Read the model definition and answer for the solid it produces. Units are mm, in the model's axes. A direction names the side the tool comes from. Give positions to 0.01 mm unless a question says otherwise; leave off trailing zeros. Write each loop counter-clockwise with the first axis right and the second up, starting at its lowest first coordinate (ties: lowest second). Pieces come first, ordered by that corner, then holes. Notation, with made-up numbers: M -38,42.25 L 9,42.25 A18 ccw 9,67.25 Z; hole C 71,38.5 d3. An arc over 180 degrees is marked long. Write each question's results on one line, items separated by ' | '. Start each with the question number.
```python
from build123d import *

# Parameters (mm, degrees)
BOTTOM_COVER_SKETCH_01_W                   = 44.37
BOTTOM_COVER_SKETCH_01_H                   = 23.06
BOTTOM_COVER_EXT_SHAPE_DEPTH               = 4.3
SALIENTE_EXTRUIR1_DEPTH                    = 1.4
CORTAR_EXTRUIR1_DEPTH                      = 30.966091253
CORTAR_EXTRUIR1_DEPTH_BACK                 = 30.966091253
VACIADO2_START                             = 0.5
VACIADO2_OUTLINE_W                         = 42.97
VACIADO2_OUTLINE_H                         = 21.06
VACIADO2_DEPTH                             = 3.8
SALIENTE_EXTRUIR2_DEPTH                    = 1.4
CORTAR_EXTRUIR2_DEPTH                      = 30.933277886
CORTAR_EXTRUIR2_DEPTH_BACK                 = 30.933277886
BOTTOM_POWER_TAKE_OFF_SHAFT_SKETCH_R       = 3
POWER_TAKE_OFF_SHAFT_EXTRUDE_01_DEPTH      = 3.9
BOTTOM_POWER_TAKE_OFF_SHAFT_SKETCH_3_R     = 4
BOTTOM_POWER_TAKE_OFF_SHAFT_SKETCH_3_R_2   = 3
POWER_TAKE_OFF_SHAFT_EXTRUDE_02_DEPTH      = 1
POWER_TAKE_OFF_SHAFT_CUT_DEPTH             = 1
POWER_TAKE_OFF_SHAFT_BOTTOM_COVER_SKETCH_R = 1
CORTAR_EXTRUIR4_DEPTH                      = 4.2
REDONDEO1_R                                = 0.5


with BuildPart() as part:
    # bottom-cover-sketch-01 → Bottom-cover-ext-shape (new body)
    with BuildSketch(Plane(origin=(0, 0, 0), x_dir=(1, 0, 0), z_dir=(0, 1, 0))):
        Rectangle(BOTTOM_COVER_SKETCH_01_W, BOTTOM_COVER_SKETCH_01_H)
    extrude(amount=BOTTOM_COVER_EXT_SHAPE_DEPTH)

    # bottom-cover-sketch-01<31> → Saliente-Extruir1 (add)
    with BuildSketch(Plane(origin=(0, 0, 0), x_dir=(1, 0, 0), z_dir=(0, 1, 0))):
        with BuildLine():
            Line((4.447, 8.15), (16.025784389, 8.15))
            ThreePointArc((16.025784389, 8.15), (17.087381076, 6.195438755), (19, 5.06001547))
            Line((19, 5.06001547), (19, -5.06001547))
            ThreePointArc((19, -5.06001547), (17.087381076, -6.195438755), (16.025784389, -8.15))
            Line((16.025784389, -8.15), (4.447, -8.15))
            Line((4.447, -8.15), (4.447, 8.15))
        make_face()
    extrude(amount=-SALIENTE_EXTRUIR1_DEPTH)

    # Croquis3 → Cortar-Extruir1 (cut, two sides: drawn at the far end of the back side and taken through both)
    with BuildSketch(Plane.XY.offset(8.15).offset(-CORTAR_EXTRUIR1_DEPTH_BACK)):
        Polygon((4.447, -1.4), (7.603, -1.4), (4.447, 0), align=None)
    extrude(amount=CORTAR_EXTRUIR1_DEPTH + CORTAR_EXTRUIR1_DEPTH_BACK, mode=Mode.SUBTRACT)

    # Vaciado2: read off the stored shape, not the designer's step
    # Vaciado2 outline → Vaciado2 (cut)
    with BuildSketch(Plane(origin=(0, 0, 0), x_dir=(1, 0, 0), z_dir=(0, 1, 0)).offset(VACIADO2_START)):
        Rectangle(VACIADO2_OUTLINE_W, VACIADO2_OUTLINE_H)
    extrude(amount=VACIADO2_DEPTH, mode=Mode.SUBTRACT)

    # Vaciado2 2: loft between two sections, ruled curve by curve
    vaciado2_2_from = [
        Edge.make_three_point_arc((15.297011486, -0.5, -7.15), (16.377210633, -0.5, -5.491282779), (18, -0.5, -4.357824492)),
        Edge.make_three_point_arc((18, -0.5, 4.357824492), (16.377210633, -0.5, 5.491282779), (15.297011486, -0.5, 7.15)),
        Edge.make_line((8.040274257, -0.5, -7.15), (15.297011486, -0.5, -7.15)),
        Edge.make_line((15.297011486, -0.5, 7.15), (8.040274257, -0.5, 7.15)),
        Edge.make_line((18, -0.5, -4.357824492), (18, -0.5, 4.357824492)),
        Edge.make_line((8.040274257, -0.5, 7.15), (8.040274257, -0.5, -7.15)),
    ]
    vaciado2_2_to = [
        Edge.make_three_point_arc((15.297011486, 0.5, -7.15), (16.377210633, 0.5, -5.491282779), (18, 0.5, -4.357824492)),
        Edge.make_three_point_arc((18, 0.5, 4.357824492), (16.377210633, 0.5, 5.491282779), (15.297011486, 0.5, 7.15)),
        Edge.make_line((5.785988543, 0.5, -7.15), (15.297011486, 0.5, -7.15)),
        Edge.make_line((15.297011486, 0.5, 7.15), (5.785988543, 0.5, 7.15)),
        Edge.make_line((18, 0.5, -4.357824492), (18, 0.5, 4.357824492)),
        Edge.make_line((5.785988543, 0.5, 7.15), (5.785988543, 0.5, -7.15)),
    ]
    vaciado2_2 = Solid(Shell([*[Face.make_surface_from_curves(vaciado2_2_from[k], vaciado2_2_to[k]) for k in range(6)], Face(Wire(vaciado2_2_from)), Face(Wire(vaciado2_2_to))]))
    add(vaciado2_2, mode=Mode.SUBTRACT)

    # bottom-cover-sketch-01<32> → Saliente-Extruir2 (add)
    with BuildSketch(Plane(origin=(0, 0, 0), x_dir=(1, 0, 0), z_dir=(0, 1, 0))):
        with BuildLine():
            Line((-1.8, -8.085967922), (-15.968544519, -8.085967922))
            ThreePointArc((-15.968544519, -8.085967922), (-17.060455349, -6.121867553), (-19, -4.986911136))
            Line((-19, -4.986911136), (-19, 5.04796656))
            ThreePointArc((-19, 5.04796656), (-17.09705221, 6.168745986), (-16.025784389, 8.1))
            Line((-16.025784389, 8.1), (-1.8, 8.1))
            Line((-1.8, 8.1), (-1.8, -8.085967922))
        make_face()
    extrude(amount=-SALIENTE_EXTRUIR2_DEPTH)

    # Croquis4 → Cortar-Extruir2 (cut, two sides: drawn at the far end of the back side and taken through both)
    with BuildSketch(Plane(origin=(0, 0, -8.1), x_dir=(-1, 0, 0), z_dir=(0, 0, -1)).offset(-CORTAR_EXTRUIR2_DEPTH_BACK)):
        Polygon((1.8, -1.4), (4.8, -1.4), (1.8, 0), align=None)
    extrude(amount=CORTAR_EXTRUIR2_DEPTH + CORTAR_EXTRUIR2_DEPTH_BACK, mode=Mode.SUBTRACT)

    # Bottom-power-take-off-shaft-sketch → Power-take-off-shaft-extrude-01 (add)
    with BuildSketch(Plane.XZ.offset(1.4)):
        with Locations(Location((-11.9, -0.018771875, 0), (0, 0, 270))):
            Circle(BOTTOM_POWER_TAKE_OFF_SHAFT_SKETCH_R)
    extrude(amount=POWER_TAKE_OFF_SHAFT_EXTRUDE_01_DEPTH)

    # Bottom-power-take-off-shaft-sketch<3> → Power-take-off-shaft-extrude-02 (add)
    with BuildSketch(Plane.XZ.offset(1.4)):
        with Locations(Location((-11.9, -0.018771875, 0), (0, 0, 90))):
            Circle(BOTTOM_POWER_TAKE_OFF_SHAFT_SKETCH_3_R)
        with Locations(Location((-11.9, -0.018771875, 0), (0, 0, 270))):
            Circle(BOTTOM_POWER_TAKE_OFF_SHAFT_SKETCH_3_R_2, mode=Mode.SUBTRACT)
    extrude(amount=POWER_TAKE_OFF_SHAFT_EXTRUDE_02_DEPTH)

    # Bottom-power-take-off-shaft-sketch<4> → Power-take-off-shaft-cut (cut)
    with BuildSketch(Plane.XZ.offset(1.4)):
        with BuildLine():
            Line((-13.454482392, -5.041059169), (-13.454482392, -6.345663941))
            ThreePointArc((-13.454482392, -6.345663941), (-13.609767702, -6.653654843), (-13.949729169, -6.711948276))
            ThreePointArc((-13.949729169, -6.711948276), (-16.710183373, -5.104254736), (-18.468864278, -2.437453767))
            ThreePointArc((-18.468864278, -2.437453767), (-18.423589426, -2.085954505), (-18.109382928, -1.922016039))
            Line((-18.109382928, -1.922016039), (-16.773422083, -1.922016039))
            ThreePointArc((-16.773422083, -1.922016039), (-16.567971503, -1.981769919), (-16.426615215, -2.142390177))
            ThreePointArc((-16.426615215, -2.142390177), (-15.30881206, -3.676640153), (-13.699675431, -4.68365862))
            ThreePointArc((-13.699675431, -4.68365862), (-13.521673241, -4.824348083), (-13.454482392, -5.041059169))
        make_face()
        with BuildLine():
            ThreePointArc((-18.070283639, 1.987983961), (-18.386311386, 2.15455721), (-18.427501404, 2.509414316))
            ThreePointArc((-18.427501404, 2.509414316), (-16.667494828, 5.106751812), (-13.949729169, 6.674404526))
            ThreePointArc((-13.949729169, 6.674404526), (-13.609767702, 6.616111093), (-13.454482392, 6.30812019))
            Line((-13.454482392, 6.30812019), (-13.454482392, 5.003515418))
            ThreePointArc((-13.454482392, 5.003515418), (-13.521673241, 4.786804333), (-13.699675431, 4.64611487))
            ThreePointArc((-13.699675431, 4.64611487), (-15.269573485, 3.675273946), (-16.380250969, 2.200991908))
            ThreePointArc((-16.380250969, 2.200991908), (-16.52151792, 2.045563265), (-16.723505638, 1.987983961))
            Line((-16.723505638, 1.987983961), (-18.070283639, 1.987983961))
        make_face()
        with BuildLine():
            ThreePointArc((-5.372498596, 2.509414316), (-6.810764187, 4.78744065), (-9.002861085, 6.353557848))
            ThreePointArc((-9.002861085, 6.353557848), (-9.368785516, 6.326920146), (-9.544482392, 6.00483186))
            Line((-9.544482392, 6.00483186), (-9.544482392, 4.615622196))
            ThreePointArc((-9.544482392, 4.615622196), (-9.494125288, 4.425766238), (-9.356293346, 4.285825255))
            ThreePointArc((-9.356293346, 4.285825255), (-8.236582512, 3.384075801), (-7.419749031, 2.200991908))
            ThreePointArc((-7.419749031, 2.200991908), (-7.27848208, 2.045563265), (-7.076494362, 1.987983961))
            Line((-7.076494362, 1.987983961), (-5.729716361, 1.987983961))
            ThreePointArc((-5.729716361, 1.987983961), (-5.413688614, 2.15455721), (-5.372498596, 2.509414316))
        make_face()
        with BuildLine():
            Line((-7.026577917, -1.922016039), (-5.690617072, -1.922016039))
            ThreePointArc((-5.690617072, -1.922016039), (-5.376410574, -2.085954505), (-5.331135722, -2.437453767))
            ThreePointArc((-5.331135722, -2.437453767), (-6.770756692, -4.782264616), (-9.002861085, -6.391101599))
            ThreePointArc((-9.002861085, -6.391101599), (-9.368785516, -6.364463896), (-9.544482392, -6.04237561))
            Line((-9.544482392, -6.04237561), (-9.544482392, -4.653165946))
            ThreePointArc((-9.544482392, -4.653165946), (-9.494125288, -4.463309988), (-9.356293346, -4.323369006))
            ThreePointArc((-9.356293346, -4.323369006), (-8.200468949, -3.382322083), (-7.373384785, -2.142390177))
            ThreePointArc((-7.373384785, -2.142390177), (-7.232028497, -1.981769919), (-7.026577917, -1.922016039))
        make_face()
    extrude(amount=-POWER_TAKE_OFF_SHAFT_CUT_DEPTH, mode=Mode.SUBTRACT)

    # Power-take-off-shaft-bottom-cover-sketch → Cortar-Extruir4 (cut)
    with BuildSketch(Plane.XZ.offset(5.3)):
        with Locations(Location((-11.9, -0.018771875, 0), (0, 0, 270))):
            Circle(POWER_TAKE_OFF_SHAFT_BOTTOM_COVER_SKETCH_R)
    extrude(amount=-CORTAR_EXTRUIR4_DEPTH, mode=Mode.SUBTRACT)

    # Redondeo1
    redondeo1_edges = [part.edges().sort_by_distance(p)[0] for p in [
        (0, 0, -11.53),
        (22.185, 0, 0),
        (0, 0, 11.53),
        (-22.185, 0, 0),
        (-22.185, 2.15, -11.53),
        (22.185, 2.15, -11.53),
        (22.185, 2.15, 11.53),
        (-22.185, 2.15, 11.53),
    ]]
    fillet(redondeo1_edges, radius=REDONDEO1_R)


solid = part.part
```
Item 1: For faces 1 (the flat face through (19, -1, 0)), 2 (the flat face through (-9, -1, -8.1)), 3 (the flat face through (0, 2, -10.53)), 4 (the flat face through (-19, -1, 0)), 5 (the flat face through (-12, -1.1, 0)), determine the directions among +Z, -Z, +X, -X, +Y, -Y from which every point of the face is accessible in a straight line to the end or side of a thin tool.
Item 2: Section C-C, the plane x = -3 is taken. Determine the outline of the cut face in (y, z).
Item 3: Determine the mould class of faces 6 (the flat face through (-10, -1.4, -4)), 7 (the flat face through (-22.185, 2, 0)), 8 (the cylindrical face through (-6.74, -0.91, -4.75)) for opening direction X: +X half, -X half, draft (parallel to the pull), parting line (faces both ways), or undercut.
Item 4: Given P1, Ø3, axis at x = 12.5, z = -3.5, coming from the +Y side; P2, Ø1.8, axis at x = -11.9, z = -0.02, coming from the +Y side; P3, Ø1.4, axis at x = -15, z = -4, coming from the -Y side, each flat-ended and moving along its own axis, determine where each tip first touches the part or whether it passes through.
Item 5: Straight lines are drawn through the part: line 1 (Z direction, x = -13.5, y = 3.25); line 2 (X direction, y = 2.5, z = -5.25) (3 decimals); line 3 (X direction, y = -0.25, z = -4.25). For each, find the intervals that lie inside material, in ascending order.
Item 6: Section B-B, the plane x = -11.9 is taken. Determine the outline of the cut face in (y, z).
Item 7: Section A-A, the plane y = 3 is taken. Determine the outline of the cut face in (x, z) (3 decimals).
Worked out:
1) face 1: +Z, -Z, +X, -Y | face 2: -Z, -X, -Y | face 3: +Y | face 4: +Z, -Z, -X, -Y | face 5: -Y
2) outline: M -0.56,-8.1 L 0,-8.1 L 0,-11.03 A0.5 ccw 0.5,-11.53 L 4.3,-11.53 L 4.3,-10.53 L 0.5,-10.53 L 0.5,10.53 L 4.3,10.53 L 4.3,11.53 L 0.5,11.53 A0.5 ccw 0,11.03 L 0,8.09 L -0.56,8.09 Z
3) face 6: draft | face 7: -X half | face 8: undercut
4) P1: stops at y = -0.5 | P2: stops at y = 0.5 | P3: stops at y = -1.4
5) line 1: z = -11.53 to -10.53, 10.53 to 11.53 | line 2: x = -22.185 to -21.485, 21.485 to 22.185 | line 3: x = -19 to -2.34, 5.01 to 7.48, 18 to 19
6) outline: M -5.3,-3.02 L -2.4,-3.02 L -2.4,-4.02 L -1.4,-4.02 L -1.4,-8.1 L 0,-8.1 L 0,-11.03 A0.5 ccw 0.5,-11.53 L 4.3,-11.53 L 4.3,-10.53 L 0.5,-10.53 L 0.5,10.53 L 4.3,10.53 L 4.3,11.53 L 0.5,11.53 A0.5 ccw 0,11.03 L 0,8.09 L -1.4,8.09 L -1.4,3.98 L -2.4,3.98 L -2.4,2.98 L -5.3,2.98 L -5.3,0.98 L -1.1,0.98 L -1.1,-1.02 L -5.3,-1.02 Z
7) outline: M -22.185,-11.03 A0.5 ccw -21.685,-11.53 L 21.685,-11.53 A0.5 ccw 22.185,-11.03 L 22.185,11.03 A0.5 ccw 21.685,11.53 L -21.685,11.53 A0.5 ccw -22.185,11.03 Z; hole M -21.485,-10.53 L 21.485,-10.53 L 21.485,10.53 L -21.485,10.53 Z
